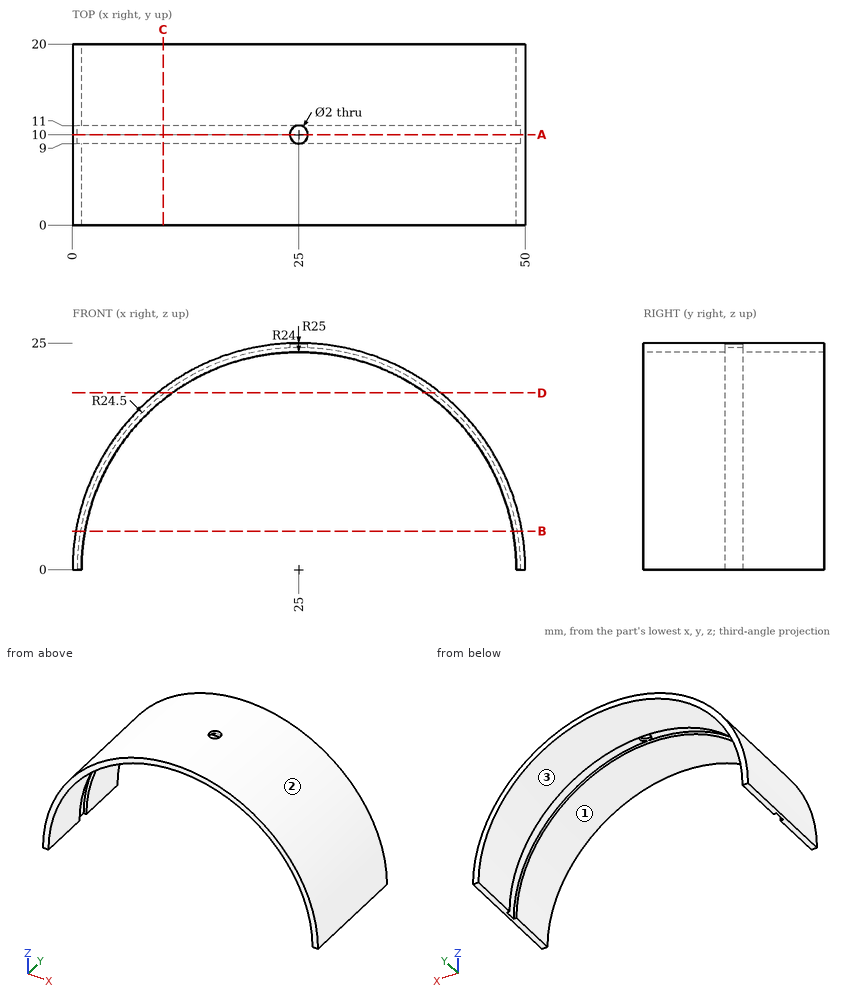
Geometry: see drawing. Coordinates: mm, zero at the bounding-box minimum. Coordinates: 2 decimals unless noted, no trailing zeros. Loops run counter-clockwise (first coordinate to the right, second up) from the corner with the lowest first, then second, coordinate; pieces in that order, holes last. Notation, with made-up numbers: (82.25, -23) - (91.25, -23) arc R32 cw to (91.25, 16) - close; hole circle Ø9 at (27, -30). An arc over 180 degrees is marked (long way). Answer in a Markdown table with one row per item.
(1) Cut plane B-B on z = 4.25. Output: boundary loops of the cut face in (x, y).
Model answer:
| item | result |
|---|---|
| outline | (0.36, 0) - (1.38, 0) - (1.38, 9) - (0.87, 9) - (0.87, 11) - (1.38, 11) - (1.38, 20) - (0.36, 20) - close; (48.62, 0) - (49.64, 0) - (49.64, 20) - (48.62, 20) - (48.62, 11) - (49.13, 11) - (49.13, 9) - (48.62, 9) - close |
(2) Cut plane D-D on z = 19.5. Output: boundary loops of the cut face in (x, y).
Model answer:
| item | result |
|---|---|
| outline | (9.36, 0) - (11.01, 0) - (11.01, 9) - (10.17, 9) - (10.17, 11) - (11.01, 11) - (11.01, 20) - (9.36, 20) - close; (38.99, 0) - (40.64, 0) - (40.64, 20) - (38.99, 20) - (38.99, 11) - (39.83, 11) - (39.83, 9) - (38.99, 9) - close |
(3) Pin query (flat end, axial travel): P1, Ø1, axis at y = 6.5, z = 3, coming from the +X side; P2, Ø12, axis at x = 42, z = 20, coming from the +Y side; P3, Ø2, axis at x = 7.5, z = 12.5, coming from the +Y side; P4, Ø3, axis at x = 14, y = 7, coming from the -Z side. Return the tip coordinate at first contact, or that it passes through.
Model answer:
| item | result |
|---|---|
| P1 | stops at x = 49.87 |
| P2 | stops at y = 20 |
| P3 | passes through |
| P4 | stops at z = 20.49 |
(4) Cut plane C-C on x = 10. Output: boundary loops of the cut face in (y, z) (3 decimals).
Model answer:
| item | result |
|---|---|
| outline | (0, 18.735) - (9, 18.735) - (9, 19.371) - (11, 19.371) - (11, 18.735) - (20, 18.735) - (20, 20) - (0, 20) - close |
(5) Mould query, pull axis X, two halves, no side actions, for the marked faces 1, 2 and 3. Classes: pulls with the +X half, pulls with the -X half, needs draft (parallel to the pull), parting line crosses it, or undercut.
Model answer:
| item | result |
|---|---|
| face 1 | undercut |
| face 2 | parting line crosses it |
| face 3 | undercut |
(6) Cut plane A-A on y = 10. Output: boundary loops of the cut face in (x, z), plus the area to 3 significant figures.
Model answer:
| item | result |
|---|---|
| outline | (0, 0) - (0.5, 0) arc R24.5 cw to (24, 24.48) - (24, 24.98) arc R25 ccw to start; (26, 24.48) arc R24.5 cw to (49.5, 0) - (50, 0) arc R25 ccw to (26, 24.98) - close |
| area | 37.9 mm² |
(7) Material intervals for L1, parallel to Y at x = 25, z = 24.75; L2, parallel to X at y = 18.5, z = 20.75; L3, parallel to X at y = 15, z = 19.5, sorted ascending. Write a range as from..to.
Model answer:
| item | result |
|---|---|
| L1 | y = 0..9, 11..20 |
| L2 | x = 11.06..12.94, 37.06..38.94 |
| L3 | x = 9.36..11.01, 38.99..40.64 |
